Autodesk Inventor part; units mm, degrees
ref_plane "YZ Plane" through (0, 0, 0) normal (1, 0, 0) x (0, 1, 0)
ref_plane "XZ Plane" through (0, 0, 0) normal (0, 1, 0) x (-1, 0, 0)
ref_plane "XY Plane" through (0, 0, 0) normal (0, 0, 1) x (1, 0, 0)
sketch "Sketch1" plane through (0, 0, 0) normal (0, 1, 0) x (-1, 0, 0)
  circle A0 centre (22.2894, -21.943) radius 11
  circle A1 centre (22.2894, -21.943) radius 7.75 construction
  circle A2 centre (22.2894, -21.943) radius 5
  circle A3 centre (22.2894, -21.943) radius 4
  point P0 (0, 0)
  point P1 (14.5394, -21.943)
  dimension "d2" = 15.5
  dimension "d1" = 22
  dimension "d4" = 10
  dimension "d17" = 8
extrude "Extrusion1" add sketch "Sketch1" along normal blind 3.5 contours A0
hole "Hole1" at (-14.5394, 0, -21.943) direction (0, 1, 0) diameter 3 end through all countersink diameter 4 countersink angle 90
pattern_circular "Circular Pattern1" count 4 over 360 about axis through (-22.2894, 0, -21.943) along (0, 1, 0) of "Hole1"
extrude "Extrusion2" add sketch "Sketch1" along normal blind 9 and the other way blind 1.5 contours A2
properties part number "ACME Brass Nut" material "Brass, Soft Yellow"
Verification items for the finished model (mm, model axes). A direction names the side the tool comes from. Coordinates: 2 decimals unless noted, no trailing zeros. Order: outer loops, then holes, each group sorted by start corner. A loop starts at its lowest first (then second) coordinate and runs counter-clockwise, first axis right, second up. Notation, with made-up numbers: (-22, 80) - (31, 80) arc R19 cw to (31, 110) - close; hole circle Ø3 at (10.5, 3). An arc over 180 degrees is marked (long way). Return JSON: item names as keys, results as strings.
(1) Section check B-B, the plane y = 2.25. Record the cut outline in (x, z).
Filled sheet:
{"outline": "circle Ø22 at (-22.29, -21.94); hole circle Ø3 at (-30.04, -21.94); hole circle Ø8 at (-22.29, -21.94); hole circle Ø3 at (-22.29, -29.69); hole circle Ø3 at (-22.29, -14.19); hole circle Ø3 at (-14.54, -21.94)"}
(2) Section check C-C, the plane x = -21.5. Give the number of separate pieces and of enclosed holes in the cut face, and give its area (3 significant figures).
Filled sheet:
{"separate pieces": "4", "enclosed holes": "0", "area": "45.1 mm^2"}
(3) Thickness scan on line 1 along X through (y, z) = (1, -23); line 2 along Y through (x, z) = (-29.5, -20); line 3 along Z through (x, y) = (-15.5, 3). Record the ranges inside material, lowest first.
Filled sheet:
{"line 1": "x = -33.24 to -31.1, -28.98 to -26.15, -18.43 to -15.6, -13.48 to -11.34", "line 2": "y = 0 to 3.5", "line 3": "z = -30.6 to -23.1, -20.79 to -13.29"}
(4) Section check D-D, the plane y = 7. Record the cut outline in (x, z), and give its area (3 significant figures).
Filled sheet:
{"outline": "circle Ø10 at (-22.29, -21.94); hole circle Ø8 at (-22.29, -21.94)", "area": "28.3 mm^2"}
(5) Go/stop test with flat-tipped pins: pin 1 (4 mm diameter, centred on x = -22, y = 0, fed in from +Z); pin 2 (1.5 mm diameter, centred on x = -18, y = 2.5, fed in from +Z); pin 3 (3 mm diameter, centred on x = -24.5, y = 1.5, fed in from -Z); pin 4 (1 mm diameter, centred on y = 6.5, z = -18.5, fed in from +X). Record where each tip stops, or that it passes through.
Filled sheet:
{"pin 1": "stops at z = -10.94", "pin 2": "stops at z = -11.53", "pin 3": "stops at z = -32.92", "pin 4": "stops at x = -18.25"}
(6) Section check A-A, the plane z = -18.25. Record the cut outline in (x, y).
Filled sheet:
{"outline": "(-32.65, 0) - (-25.66, 0) - (-25.66, -1.5) - (-23.83, -1.5) - (-23.83, 9) - (-25.66, 9) - (-25.66, 3.5) - (-32.65, 3.5) - close; (-20.75, -1.5) - (-18.92, -1.5) - (-18.92, 0) - (-11.93, 0) - (-11.93, 3.5) - (-18.92, 3.5) - (-18.92, 9) - (-20.75, 9) - close"}
(7) Access from +Z, -Z, +X, -X, +Y, -Y to the whole of each face (thin tool, end or side, straight path). Record for faces 4 (the cylindrical face through (-26.91, 6.21, -20.03)), 5 (the cylindrical face through (-20.904, 2.021, -13.618)), 6 (the cylindrical face through (-24.597, -0.74, -26.379)).
Filled sheet:
{"face 4": "+Y", "face 5": "+Y, -Y", "face 6": "-Y"}
(8) Mould release check, pull along Z, two halves, no side actions. Record for faces 1 (the flat face through (-17, 0, -22)), 2 (the cylindrical face through (-19.905, 1.726, -11.205)), 3 (the cylindrical face through (-26.105, 3.676, -23.144)): pulls with the +Z half, pulls with the -Z half, needs draft (parallel to the pull), parting line crosses it, or undercut.
Filled sheet:
{"face 1": "needs draft", "face 2": "parting line crosses it", "face 3": "undercut"}
